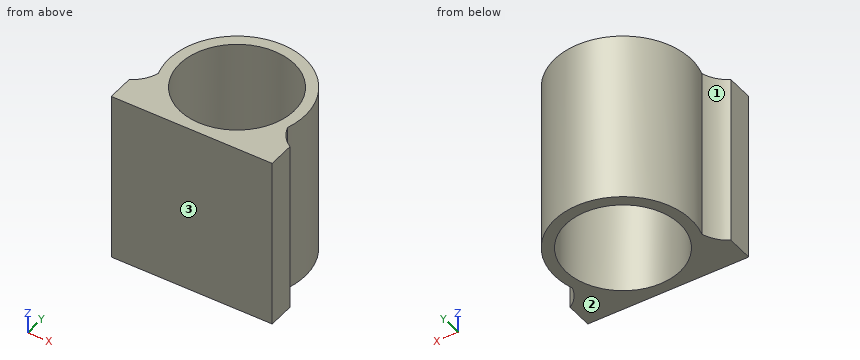
```python
from build123d import *

# Parameters (mm, degrees)
SKETCH1_R           = 18.5
SKETCH1_R_2         = 15.5
BOSS_EXTRUDE1_DEPTH = 46.6
SKETCH4_W           = 43.709561032
SKETCH4_H           = 12.768078571
BOSS_EXTRUDE2_DEPTH = 46.6
SKETCH5_R           = 15.5
CUT_EXTRUDE1_DEPTH  = 55.698893074
CUT_EXTRUDE4_DEPTH  = 46.6


# Read off the part's stored shape, not the designer's step: Cut-Extrude4
with BuildPart() as part:
    # Sketch1 → Boss-Extrude1 (new body)
    with BuildSketch(Plane.XY):
        Circle(SKETCH1_R)
        Circle(SKETCH1_R_2, mode=Mode.SUBTRACT)
    extrude(amount=BOSS_EXTRUDE1_DEPTH)

    # Sketch4 → Boss-Extrude2 (add, through all)
    with BuildSketch(Plane.XY):
        with Locations((0, -12.13021123)):
            Rectangle(SKETCH4_W, SKETCH4_H)
    extrude(amount=BOSS_EXTRUDE2_DEPTH)

    # Sketch5 → Cut-Extrude1 (cut, through all)
    with BuildSketch(Plane.XY):
        Circle(SKETCH5_R)
    extrude(amount=CUT_EXTRUDE1_DEPTH, mode=Mode.SUBTRACT)

    # Cut-Extrude4 outline → Cut-Extrude4 (cut)
    with BuildSketch(Plane.XY):
        with BuildLine():
            ThreePointArc((-21.854780516, -11.237165736), (-19.197353427, -8.897985946), (-17.584979613, -5.746171944))
            Line((-17.584979613, -5.746171944), (-21.854780516, -5.746171944))
            Line((-21.854780516, -5.746171944), (-21.854780516, -11.237165736))
        make_face()
    cut_extrude4 = extrude(amount=CUT_EXTRUDE4_DEPTH, mode=Mode.SUBTRACT)

    # Mirror2: Cut-Extrude4 across plane
    add(cut_extrude4.mirror(Plane(origin=(0, 0, 0), x_dir=(0, 0, 1), z_dir=(1, 0, 0))), mode=Mode.SUBTRACT)


solid = part.part
```
For this review, take the finished solid that the model builds, in its own axes (mm). Face numbers are marked on the shaded views. Coordinates: 2 decimals unless noted, no trailing zeros. Loops run counter-clockwise (first coordinate to the right, second up) from the corner with the lowest first, then second, coordinate; pieces in that order, holes last. Notation, with made-up numbers: (-34, 52.25) - (22, 52.25) arc R31 cw to (22, 80.25) - close; hole circle Ø7 at (44.25, 35). An arc over 180 degrees is marked (long way). Use one line per item in the form item = value. Start each with the question number.
1) Draft analysis for pull direction Y (two halves, no side actions). For the marked faces 1, 2 and 3, state which applies: released by +Y, released by -Y, zero draft, split by the parting line, or undercut.
2) Take a section at A-A (y = 0). State the section outline as (x, z) points, plus the area to 3 significant figures.
3) To check wall thickness, follow probe 1 along Y at (x, z) = (0, 10); probe 2 along X at (y, z) = (0, 32.5); probe 3 along Y at (x, z) = (-3.5, 43). State the ranges of each line that lie inside material, in increasing order. Write a range as from..to.
4) For pin 1 (2 mm diameter, centred on y = 4.5, z = 15.5, fed in from +X); pin 2 (6 mm diameter, centred on x = 1, z = 38.5, fed in from +Y); pin 3 (1 mm diameter, centred on y = -4, z = 6, fed in from -X); pin 4 (10 mm diameter, centred on x = -14.5, z = 21.5, fed in from +Y), all flat-tipped, find the tip position at first contact; note any pin that passes through.
5) Take a section at B-B (x = 3.5). State the section outline as (y, z) points, plus the area to 3 significant figures.
6) Take a section at C-C (z = 15.5). State the section outline as (x, y) points, plus the area to 3 significant figures.
From the geometry:
q1.face_1 = undercut
q1.face_2 = zero draft
q1.face_3 = released by -Y
q2.outline = (-18.5, 0) - (-15.5, 0) - (-15.5, 46.6) - (-18.5, 46.6) - close; (15.5, 0) - (18.5, 0) - (18.5, 46.6) - (15.5, 46.6) - close
q2.area = 280 mm2
q3.probe_1 = -18.51..-15.5, 15.5..18.5
q3.probe_2 = -18.5..-15.5, 15.5..18.5
q3.probe_3 = -18.51..-15.1, 15.1..18.17
q4.pin_1 = 18.17
q4.pin_2 = 18.5
q4.pin_3 = -18.17
q4.pin_4 = 15.87
q5.outline = (-18.51, 0) - (-15.1, 0) - (-15.1, 46.6) - (-18.51, 46.6) - close; (15.1, 0) - (18.17, 0) - (18.17, 46.6) - (15.1, 46.6) - close
q5.area = 302 mm2
q6.outline = (-21.85, -18.51) - (21.85, -18.51) - (21.85, -11.24) arc R9.47 cw to (17.58, -5.75) arc R18.5 ccw (long way) to (-17.58, -5.75) arc R9.47 cw to (-21.85, -11.24) - close; hole circle Ø31 at (0, 0)
q6.area = 520 mm2
